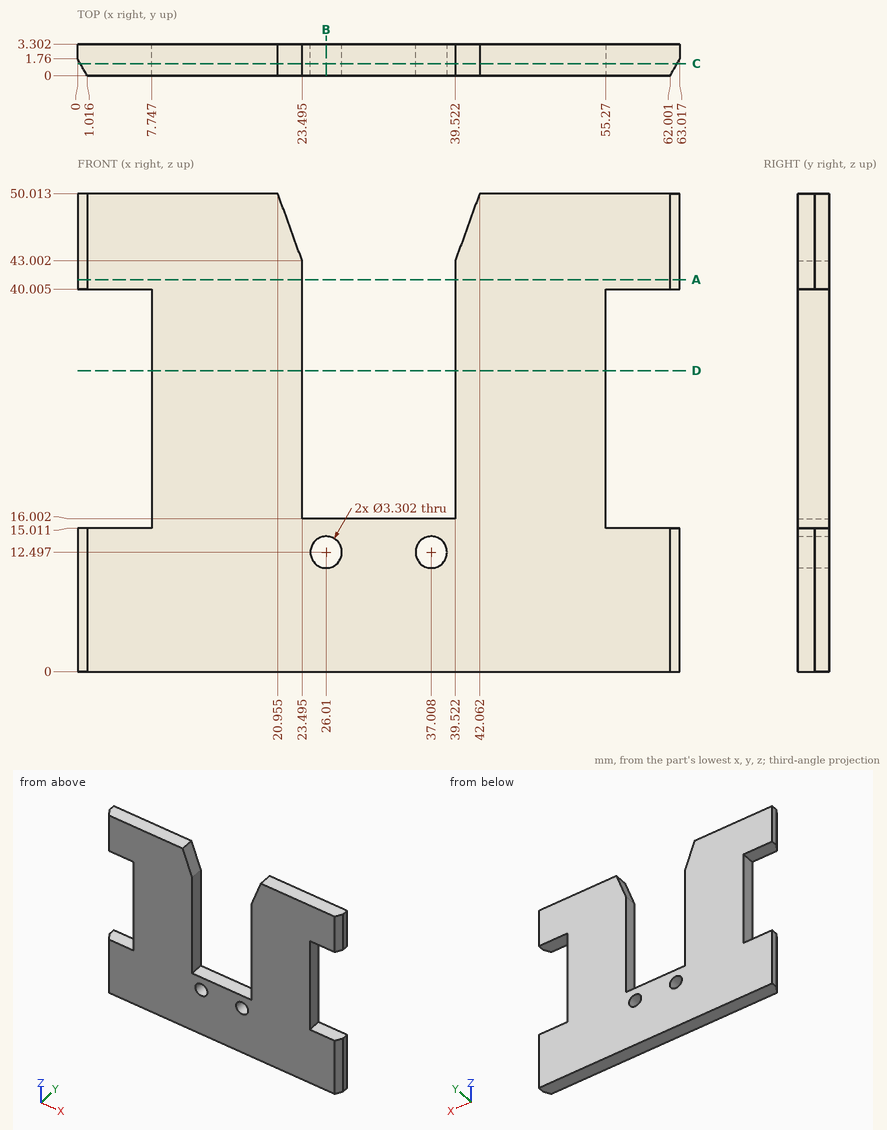
Geometry check sheet. Reference: drawing and pictorial views, mm from the part's lowest x, y, z. Coordinates: 2 decimals unless noted, no trailing zeros. Write each loop counter-clockwise with the first axis right and the second up, starting at its lowest first coordinate (ties: lowest second). Pieces come first, ordered by that corner, then holes. Notation, with made-up numbers: M 3.5,8.25 L 40.5,8.25 A27 cw 40.5,40.25 Z; hole C 25,13.25 d1. An arc over 180 degrees is marked long. Write item = value, one per line. Start each with the question number.
1. Go/stop test with flat-tipped pins: pin 1 (1.7 mm diameter, centred on y = 2, z = 23, fed in from -X); pin 2 (1 mm diameter, centred on y = 1.5, z = 35, fed in from +X). Record where each tip stops, or that it passes through.
2. Sectioned sample at D-D (z = 31.5). Record the cut outline in (x, y) (1 decimal), then the cut area to 3 significant figures.
3. Thickness scan on probe 1 along Z at (x, y) = (57, 1.6) (1 decimal); probe 2 along X at (y, z) = (2, 31.5) (1 decimal); probe 3 along Z at (x, y) = (24.5, 1.3) (1 decimal). Record the ranges inside material, lowest first.
4. Sectioned sample at B-B (x = 26). Record the cut outline in (y, z) (1 decimal).
5. Sectioned sample at C-C (y = 1.25). Record the cut outline in (x, z) (1 decimal), then the cut area to 3 significant figures.
6. Sectioned sample at A-A (z = 41). Record the cut outline in (x, y) (1 decimal).
The answers:
q1.pin_1 = 7.75
q1.pin_2 = 55.27
q2.outline = M 7.7,0 L 23.5,0 L 23.5,3.3 L 7.7,3.3 Z; M 39.5,0 L 55.3,0 L 55.3,3.3 L 39.5,3.3 Z
q2.area = 104 mm²
q3.probe_1 = 0 to 15, 40 to 50
q3.probe_2 = 7.7 to 23.5, 39.5 to 55.3
q3.probe_3 = 0 to 11.8, 13.2 to 16
q4.outline = M 0,0 L 3.3,0 L 3.3,10.8 L 0,10.8 Z; M 0,14.1 L 3.3,14.1 L 3.3,16 L 0,16 Z
q5.outline = M 0.3,0 L 62.7,0 L 62.7,15 L 55.3,15 L 55.3,40 L 62.7,40 L 62.7,50 L 42.1,50 L 39.5,43 L 39.5,16 L 23.5,16 L 23.5,43 L 21,50 L 0.3,50 L 0.3,40 L 7.7,40 L 7.7,15 L 0.3,15 Z; hole C 26,12.5 d3.3; hole C 37,12.5 d3.3
q5.area = 2,170 mm²
q6.outline = M 0,1.8 L 1,0 L 23.5,0 L 23.5,3.3 L 0,3.3 Z; M 39.5,0 L 62,0 L 63,1.8 L 63,3.3 L 39.5,3.3 Z
